Autodesk Inventor part; units mm, degrees
ref_plane "Work Plane1" through (-12, -12, -7.9972) normal (0, 0, 1) x (1, 0, 0)
ref_plane "YZ Plane" through (0, 0, 0) normal (1, 0, 0) x (0, 1, 0)
ref_plane "XZ Plane" through (0, 0, 0) normal (0, 1, 0) x (-1, 0, 0)
ref_plane "Work Plane1" through (-12, -12, -7.9972) normal (0, 0, 1) x (1, 0, 0)
sketch "Sketch1" plane through (0, 0, 0) normal (0, 0, 1) x (1, 0, 0)
  circle A0 centre (0, 0) radius 9.75
  circle A1 centre (0, 0) radius 7.5
  dimension "d0" = 19.5
  dimension "d1" = 15
extrude "Extrusion1" add sketch "Sketch1" against normal up to surface (7.9972 mm away) contours A0 | A1
extrude "Extrusion2" add sketch "Sketch1" against normal blind 15 contours A1
sketch "Sketch2" plane through (0, 0, -15) normal (0, 0, -1) x (-1, 0, 0)
  circle A0 centre (4, 0) radius 1.75
  circle A1 centre (-4, 0) radius 1.75
  point P0 (0, 0)
  dimension "d6" = 3.5
  dimension "d7" = 4
  dimension "d8" = 8
extrude "Extrusion3" cut sketch "Sketch2" against normal through all
equation "\"d8\" = 2 * d7"
properties part number "Shaft-1"
Geometry: final body of the model. Coordinates: model frame, mm. A direction names the side the tool comes from. Give positions to 0.01 mm unless a question says otherwise; leave off trailing zeros. Loops run counter-clockwise (first coordinate to the right, second up) from the corner with the lowest first, then second, coordinate; pieces in that order, holes last. Notation, with made-up numbers: M -28.5,19 L -16.5,19 A16 cw -16.5,47 Z; hole C 65,-7.5 d4. An arc over 180 degrees is marked long. Put each result on its own line as item: value. Start each with the question number.
1) Contact query for flat-ended pins moving along their axis: pin 1 (5 mm diameter, centred on x = 6.5, z = -9, fed in from -Y); pin 2 (2 mm diameter, centred on y = -5, z = -10, fed in from +X). Output: stop coordinate, or through.
2) Pull-direction query (Y, two-part tool) for faces 3 (the cylindrical face through (5.75, 0.08, -7.6)), 4 (the cylindrical face through (-1.269, 9.667, -3.943)), 5 (the flat face through (0, 0, -15)); classes: pulls with the +Y half, pulls with the -Y half, needs draft (parallel to the pull), parting line crosses it, or undercut.
3) Cut plane A-A (y = 0). Output: boundary loops of the cut face in (x, z), then the cut area to 3 significant figures.
4) Cut plane B-B (x = 4). Output: boundary loops of the cut face in (y, z), then the cut area to 3 significant figures.
5) Cut plane C-C (x = 0). Output: boundary loops of the cut face in (y, z).
6) Access query for faces 1 (the cylindrical face through (-7.493, 0.33, -11.45)), 2 (the cylindrical face through (-2.25, 0.08, -7.6)). Directions: +Z, -Z, +X, -X, +Y, -Y. A direction counts if a zero-diameter tool reaches every point of the face in a straight line with its end or side. Return the directions, or none.
7) Cut plane D-D (z = -13.25). Output: boundary loops of the cut face in (x, y), then the cut area to 3 significant figures.
8) Ray query, line 1 along Y through (x, z) = (-4, -11.5); line 2 along Z through (x, y) = (-8, -4.25); line 3 along Y through (x, z) = (2.5, -6). Return the intervals inside material, ascending.
Verdict:
1. pin 1: y = -8.79
1. pin 2: x = 6.34
2. face 3: undercut
2. face 4: parting line crosses it
2. face 5: needs draft
3. outline: M -9.75,-8 L -7.5,-8 L -7.5,-15 L -5.75,-15 L -5.75,0 L -9.75,0 Z; M -2.25,-15 L 2.25,-15 L 2.25,0 L -2.25,0 Z; M 5.75,-15 L 7.5,-15 L 7.5,-8 L 9.75,-8 L 9.75,0 L 5.75,0 Z
3. area: 156 mm2
4. outline: M -8.89,-8 L -6.34,-8 L -6.34,-15 L -1.75,-15 L -1.75,0 L -8.89,0 Z; M 1.75,-15 L 6.34,-15 L 6.34,-8 L 8.89,-8 L 8.89,0 L 1.75,0 Z
4. area: 179 mm2
5. outline: M -9.75,-8 L -7.5,-8 L -7.5,-15 L 7.5,-15 L 7.5,-8 L 9.75,-8 L 9.75,0 L -9.75,0 Z
6. face 1: -Z
6. face 2: +Z, -Z
7. outline: C 0,0 d15; hole C -4,0 d3.5; hole C 4,0 d3.5
7. area: 157 mm2
8. line 1: -6.34 to -1.75, 1.75 to 6.34
8. line 2: -8 to 0
8. line 3: -9.42 to -0.9, 0.9 to 9.42
